Geometry check sheet. Reference: drawing and pictorial views, mm from the part's lowest x, y, z. A direction names the side the tool comes from. Give positions to 0.01 mm unless a question says otherwise; leave off trailing zeros. Loops run counter-clockwise (first coordinate to the right, second up) from the corner with the lowest first, then second, coordinate; pieces in that order, holes last. Notation, with made-up numbers: (21.25, -21) - (45.25, -21) arc R11 cw to (45.25, -17) - close; hole circle Ø2 at (42.25, 48). An arc over 180 degrees is marked (long way). One line per question, with ' | ' between items. Start each with the question number.
1. Depth check by flat-ended pin: pin 1 Ø8 at (y, z) = (8, 118.5) entering from -X; pin 2 Ø12 at (x, y) = (99.5, 12.5) entering from -Z; pin 3 Ø5 at (y, z) = (6.5, 39.5) entering from +X. Enter the tip coordinate at first touch or a pass-through.
2. Section check D-D, the plane x = 51.5. Enter the section's corners in (y, z).
3. Section check B-B, the plane y = 20. Enter the section's corners in (x, z), then the cut area to 3 significant figures.
4. Thickness scan on line 1 along X through (y, z) = (28.1, 94); line 2 along Z through (x, y) = (84, 1.6); line 3 along Y through (x, z) = (42, 156). Record the ranges inside material, lowest first. Write a range as from..to.
5. Tool access check on the marked faces 1 and 2. Record the directions out of +Z, -Z, +X, -X, +Y, -Y that give a thin tool (end or side, any length) a straight path to the whole face; none if there is none.
6. Section check C-C, the plane z = 64. Enter the section's corners in (x, y), then the cut area to 3 significant figures.
7. Section check A-A, the plane z = 84. Enter the section's corners in (x, y), then the cut area to 3 significant figures.
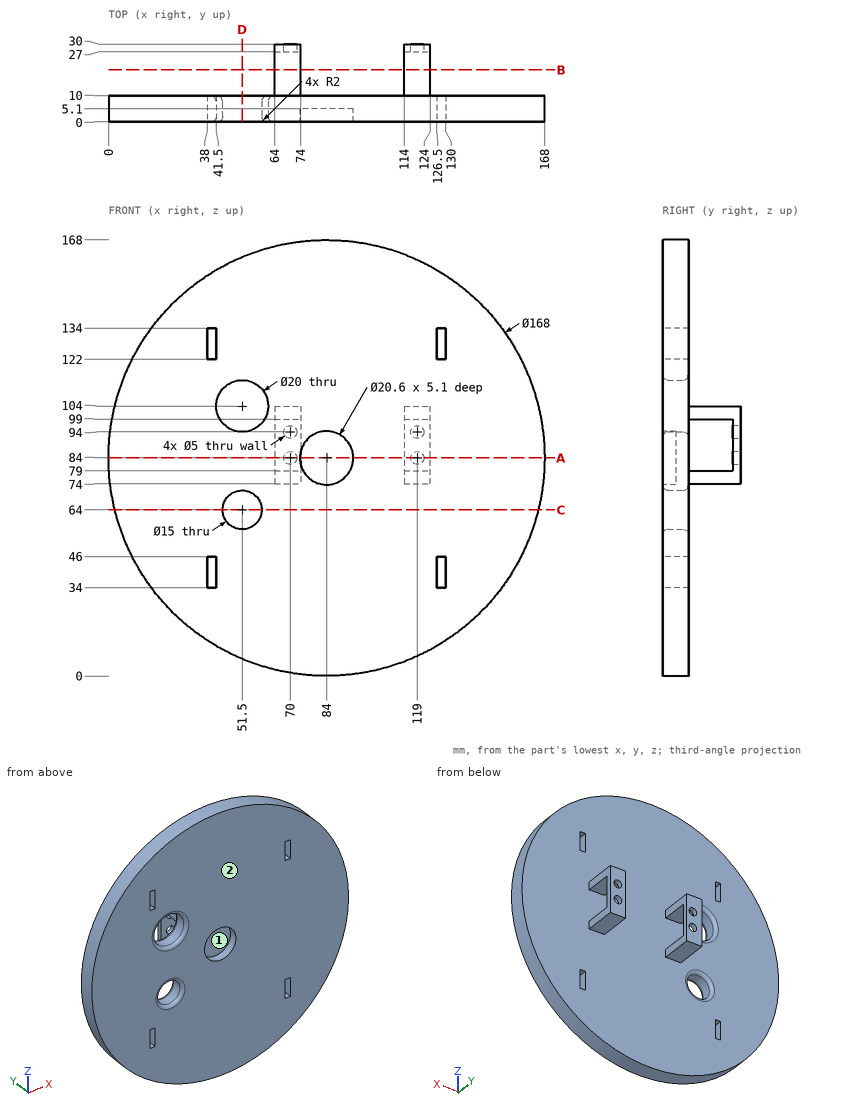
Results list:
1) pin 1: x = 5.73 | pin 2: z = 0.6 | pin 3: x = 156.75
2) outline: (0, 6.54) - (10, 6.54) - (10, 54.5) arc R2 ccw to (8, 56.5) - (2, 56.5) arc R2 ccw to (0, 54.5) - close; (0, 73.5) arc R2 ccw to (2, 71.5) - (8, 71.5) arc R2 ccw to (10, 73.5) - (10, 92) arc R2 ccw to (8, 94) - (2, 94) arc R2 ccw to (0, 92) - close; (0, 116) arc R2 ccw to (2, 114) - (8, 114) arc R2 ccw to (10, 116) - (10, 161.46) - (0, 161.46) - close
3) outline: (64, 74) - (74, 74) - (74, 79) - (64, 79) - close; (64, 99) - (74, 99) - (74, 104) - (64, 104) - close; (114, 74) - (124, 74) - (124, 79) - (114, 79) - close; (114, 99) - (124, 99) - (124, 104) - (114, 104) - close | area: 200 mm²
4) line 1: 64..67.5, 72.5..74, 114..116.5, 121.5..124 | line 2: 0..73.7, 94.3..168 | line 3: 0..10
5) face 1: -Y | face 2: +Z, -Z, +X, -X, -Y
6) outline: (2.42, 0) - (42, 0) arc R2 ccw to (44, 2) - (44, 8) arc R2 ccw to (42, 10) - (2.42, 10) - close; (59, 2) arc R2 ccw to (61, 0) - (165.58, 0) - (165.58, 10) - (61, 10) arc R2 ccw to (59, 8) - close | area: 1,480 mm²
7) outline: (0, 0) - (73.7, 0) - (73.7, 5.1) - (94.3, 5.1) - (94.3, 0) - (168, 0) - (168, 10) - (0, 10) - close; (64, 27) - (67.5, 27) - (67.5, 30) - (64, 30) - close; (72.5, 27) - (74, 27) - (74, 30) - (72.5, 30) - close; (114, 27) - (116.5, 27) - (116.5, 30) - (114, 30) - close; (121.5, 27) - (124, 27) - (124, 30) - (121.5, 30) - close | area: 1,600 mm²
